```python
from build123d import *

# Parameters (mm, degrees)
SKETCH1_W           = 80
SKETCH1_H           = 80
BOSS_EXTRUDE1_DEPTH = 900
SHELL1_T            = -3
SKETCH2_W           = 150
SKETCH2_H           = 150
SKETCH2_R           = 4
BOSS_EXTRUDE2_DEPTH = 3
SKETCH6_W           = 150
SKETCH6_H           = 80
BOSS_EXTRUDE4_DEPTH = 3
CUT_EXTRUDE3_REACH  = 914.187
SKETCH7_R           = 4
BOSS_EXTRUDE5_DEPTH = 1.5


with BuildPart() as part:
    # Sketch1 → Boss-Extrude1 (new body)
    with BuildSketch(Plane.XY):
        Rectangle(SKETCH1_W, SKETCH1_H)
    extrude(amount=BOSS_EXTRUDE1_DEPTH)

    # Shell1
    shell1_openings = [part.faces().sort_by_distance(p)[0] for p in [
        (0, 0, 900),
        (0, 0, 0),
    ]]
    offset(amount=SHELL1_T, openings=shell1_openings, kind=Kind.INTERSECTION)

    # Sketch2 → Boss-Extrude2 (add)
    with BuildSketch(Plane(origin=(0, 0, 0), x_dir=(-1, 0, 0), z_dir=(0, 0, -1))):
        Rectangle(SKETCH2_W, SKETCH2_H)
        with Locations((50, 50)):
            Circle(SKETCH2_R, mode=Mode.SUBTRACT)
        with Locations(Location((-50, 50, 0), (0, 0, 180))):
            Circle(SKETCH2_R, mode=Mode.SUBTRACT)
        with Locations(Location((50, -50, 0), (0, 0, 180))):
            Circle(SKETCH2_R, mode=Mode.SUBTRACT)
        with Locations((-50, -50)):
            Circle(SKETCH2_R, mode=Mode.SUBTRACT)
    extrude(amount=BOSS_EXTRUDE2_DEPTH)

    # Sketch6 → Boss-Extrude4 (add)
    with BuildSketch(Plane.XY.offset(900)):
        Rectangle(SKETCH6_W, SKETCH6_H)
    extrude(amount=BOSS_EXTRUDE4_DEPTH)

    # Sketch7 → Cut-Extrude3 (cut, up to next)
    with BuildSketch(Plane.XY.offset(903), mode=Mode.PRIVATE) as cut_extrude3_sk1:
        with Locations((-60, 25)):
            Circle(SKETCH7_R)
    cut_extrude3_tool1 = extrude(cut_extrude3_sk1.sketch, amount=-CUT_EXTRUDE3_REACH, mode=Mode.PRIVATE) & part.part
    # Sketch7 → Cut-Extrude3 (cut, up to next)
    with BuildSketch(Plane.XY.offset(903), mode=Mode.PRIVATE) as cut_extrude3_sk2:
        with Locations((60, 25)):
            Circle(SKETCH7_R)
    cut_extrude3_tool2 = extrude(cut_extrude3_sk2.sketch, amount=-CUT_EXTRUDE3_REACH, mode=Mode.PRIVATE) & part.part
    # Sketch7 → Cut-Extrude3 (cut, up to next)
    with BuildSketch(Plane.XY.offset(903), mode=Mode.PRIVATE) as cut_extrude3_sk3:
        with Locations((60, -25)):
            Circle(SKETCH7_R)
    cut_extrude3_tool3 = extrude(cut_extrude3_sk3.sketch, amount=-CUT_EXTRUDE3_REACH, mode=Mode.PRIVATE) & part.part
    # Sketch7 → Cut-Extrude3 (cut, up to next)
    with BuildSketch(Plane.XY.offset(903), mode=Mode.PRIVATE) as cut_extrude3_sk4:
        with Locations((-60, -25)):
            Circle(SKETCH7_R)
    cut_extrude3_tool4 = extrude(cut_extrude3_sk4.sketch, amount=-CUT_EXTRUDE3_REACH, mode=Mode.PRIVATE) & part.part
    add(cut_extrude3_tool1.solids().sort_by_distance((-60, 25, 903))[0], mode=Mode.SUBTRACT)
    add(cut_extrude3_tool2.solids().sort_by_distance((60, 25, 903))[0], mode=Mode.SUBTRACT)
    add(cut_extrude3_tool3.solids().sort_by_distance((60, -25, 903))[0], mode=Mode.SUBTRACT)
    add(cut_extrude3_tool4.solids().sort_by_distance((-60, -25, 903))[0], mode=Mode.SUBTRACT)

    # Sketch10 → Boss-Extrude5 (add, symmetric)
    with BuildSketch(Plane(origin=(0, 0, 0), x_dir=(1, 0, 0), z_dir=(0, 1, 0))):
        Polygon((-40, -900), (-75, -900), (-40, -865), align=None)
    boss_extrude5 = extrude(amount=BOSS_EXTRUDE5_DEPTH, both=True)

    # Mirror3: Boss-Extrude5 across plane
    add(boss_extrude5.mirror(Plane(origin=(0, 0, 0), x_dir=(0, 0, 1), z_dir=(1, 0, 0))))


solid = part.part
```
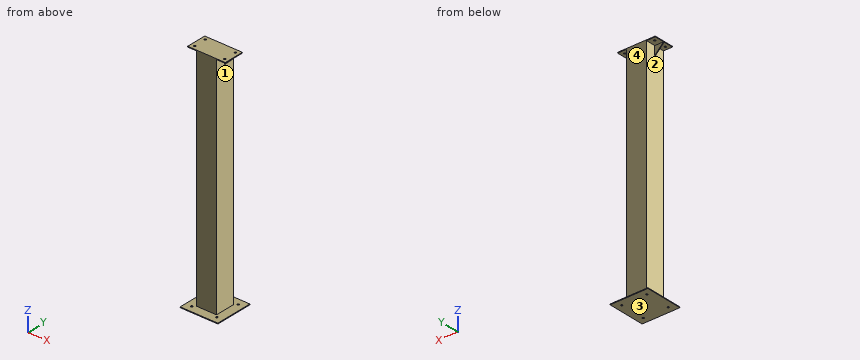
Read the model definition and answer for the solid it produces. Units are mm, in the model's axes. Face numbers are marked on the shaded views. Coordinates: 2 decimals unless noted, no trailing zeros. Loops run counter-clockwise (first coordinate to the right, second up) from the corner with the lowest first, then second, coordinate; pieces in that order, holes last. Notation, with made-up numbers: (83.25, 79) - (134.25, 79) arc R24 ccw to (134.25, 104) - close; hole circle Ø7 at (-5, -37.75). An arc over 180 degrees is marked (long way). Answer in a Markdown table with one row per item.
1. Determine the mould class of the marked faces 1, 2, 3 and 4 for opening direction Z: +Z half, -Z half, draft (parallel to the pull), parting line (faces both ways), or undercut.
Conclusion:
| item | result |
|---|---|
| face 1 | undercut |
| face 2 | undercut |
| face 3 | -Z half |
| face 4 | draft |
2. Find section B-B, the plane x = 20. Write down the section's boundary in (y, z), then the cut area to 3 significant figures.
Conclusion:
| item | result |
|---|---|
| outline | (-75, -3) - (75, -3) - (75, 0) - (40, 0) - (40, 903) - (-40, 903) - (-40, 0) - (-75, 0) - close; hole (-37, 0) - (37, 0) - (37, 900) - (-37, 900) - close |
| area | 6,090 mm² |
3. Find section C-C, the plane y = -64. Write down the section's boundary in (x, z).
Conclusion:
| item | result |
|---|---|
| outline | (-75, -3) - (75, -3) - (75, 0) - (-75, 0) - close |
4. Straight lines are drawn through the part: line 1 (Y direction, x = -50, z = -1.25); line 2 (Y direction, x = -60, z = 901); line 3 (Z direction, x = -30.5, y = 32). For each, find the intervals that lie inside material, in ascending order.
Conclusion:
| item | result |
|---|---|
| line 1 | y = -75 to -54, -46 to 46, 54 to 75 |
| line 2 | y = -40 to -29, -21 to 21, 29 to 40 |
| line 3 | z = -3 to 0, 900 to 903 |
5. Given pin 1 (10.5 mm diameter, centred on x = 52, z = 880.5, fed in from +Y); pin 2 (2 mm diameter, centred on x = -23.5, z = 219, fed in from +Y); pin 3 (1.5 mm diameter, centred on x = -25, z = 288, fed in from -Y), each flat-ended and moving along its own axis, determine where each tip first touches the part or whether it passes through.
Conclusion:
| item | result |
|---|---|
| pin 1 | stops at y = 1.5 |
| pin 2 | stops at y = 40 |
| pin 3 | stops at y = -40 |
6. Find section A-A, the plane z = 522.5. Write down the section's boundary in (x, y), then the cut area to 3 significant figures.
Conclusion:
| item | result |
|---|---|
| outline | (-40, -40) - (40, -40) - (40, 40) - (-40, 40) - close; hole (-37, -37) - (37, -37) - (37, 37) - (-37, 37) - close |
| area | 924 mm² |
